Autodesk Inventor part; units mm, degrees
ref_plane "YZ Plane" through (0, 0, 0) normal (1, 0, 0) x (0, 1, 0)
ref_plane "XZ Plane" through (0, 0, 0) normal (0, 1, 0) x (-1, 0, 0)
ref_plane "XY Plane" through (0, 0, 0) normal (0, 0, 1) x (1, 0, 0)
sketch "Sketch3" plane through (0, 0, 0) normal (0, 0, 1) x (1, 0, 0)
  line L0 (735, 1100) -> (735, 35.3553)
  line L1 (735, 35.3553) -> (699.6447, 0)
  line L2 (699.6447, 0) -> (-699.6447, 0)
  line L3 (-699.6447, 0) -> (-735, 35.3553)
  line L4 (-735, 35.3553) -> (-735, 1100)
  line L5 (-735, 1100) -> (735, 1100)
  line L6 (0, 0) -> (0, 1100) construction
  line L7 (675, 1100) -> (584.0074, 850)
  line L8 (584.0074, 850) -> (159.0074, 850)
  line L9 (159.0074, 850) -> (68.0149, 1100)
  line L10 (-68.0149, 1100) -> (-159.0074, 850)
  line L11 (-159.0074, 850) -> (-584.0074, 850)
  line L12 (-584.0074, 850) -> (-675, 1100)
  line L13 (-735, 35.3553) -> (-735, 0)
  line L14 (-735, 0) -> (-699.6447, 0)
  line L15 (699.6447, 0) -> (735, 0)
  line L16 (735, 0) -> (735, 35.3553)
  dimension "d25" = 50
  dimension "d26" = 1100
  dimension "d27" = 1470
  dimension "d32" = 425
  dimension "d33" = 60
  dimension "d35" = 250
  dimension "d38" = 110
extrude "Plate3" add sketch "Sketch3" along normal blind 2 contours L0 L1 L2 L3 L4 L5 L12 L11 L10 L9 L8 L7 | L16 L15 L1 | L14 L13 L3
equation "\"d28\" = Thickness"
equation "\"BendRadius\" = Thickness"
equation "\"BendReliefWidth\" = Thickness"
equation "\"BendReliefDepth\" = 0.5 * Thickness"
equation "\"CornerReliefSize\" = 4 * Thickness"
equation "\"MinimumRemnant\" = 2 * Thickness"
equation "\"TransitionRadius\" = BendRadius"
equation "\"JacobiRadiusSize\" = BendRadius"
equation "\"GapSize\" = Thickness"
properties part number "GBK-RK-0015 partition 5"
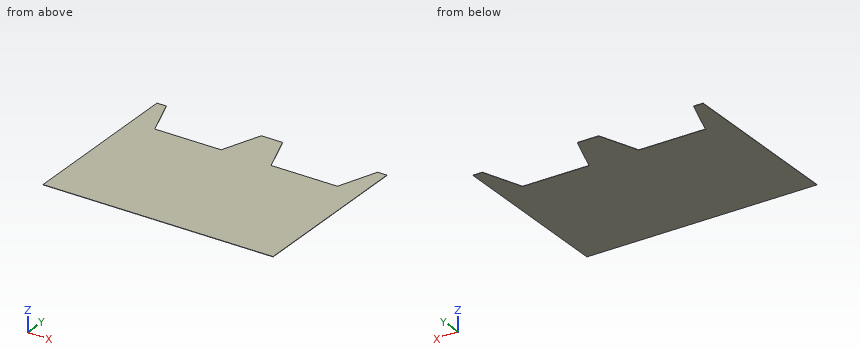
The listing builds one solid part. Answer for the finished solid, in the listing's coordinates (mm). Coordinates: 2 decimals unless noted, no trailing zeros. Write each loop counter-clockwise with the first axis right and the second up, starting at its lowest first coordinate (ties: lowest second). Pieces come first, ordered by that corner, then holes. Notation, with made-up numbers: (53.5, 18.25) - (107.5, 18.25) arc R17 cw to (107.5, 31.25) - close; hole circle Ø1 at (77.25, 60). An arc over 180 degrees is marked (long way). Return JSON: item names as keys, results as strings. Group by question number.
1. A cutting plane is placed at C-C, the plane x = 238. Determine the outline of the cut face in (y, z).
2. Given pin 1 (0.6 mm diameter, centred on x = 321.5, z = 0.5, fed in from +Y), flat-ended and moving along its own axis, determine where the tip first touches the part or whether it passes through.
3. Straight lines are drawn through the part: L1, parallel to X at y = 999, z = 1.4; L2, parallel to X at y = 902.5, z = 1.4; L3, parallel to Y at x = 339, z = 1.5. For each, find the intervals that lie inside material, in ascending order.
4. A cutting plane is placed at A-A, the plane z = 0.7. Determine the outline of the cut face in (x, y), plus the area to 3 significant figures.
5. A cutting plane is placed at B-B, the plane y = 872.5. Determine the outline of the cut face in (x, z).
Ans:
{
 "1": {"outline": "(0, 0) - (850, 0) - (850, 2) - (0, 2) - close"},
 "2": {"pin 1": "y = 850"},
 "3": {"L1": "-735 to -638.24, -104.78 to 104.78, 638.24 to 735", "L2": "-735 to -603.12, -139.9 to 139.9, 603.12 to 735", "L3": "0 to 850"},
 "4": {"outline": "(-735, 0) - (735, 0) - (735, 1100) - (675, 1100) - (584.01, 850) - (159.01, 850) - (68.01, 1100) - (-68.01, 1100) - (-159.01, 850) - (-584.01, 850) - (-675, 1100) - (-735, 1100) - close", "area": "1,360,000 mm²"},
 "5": {"outline": "(-735, 0) - (-592.2, 0) - (-592.2, 2) - (-735, 2) - close; (-150.82, 0) - (150.82, 0) - (150.82, 2) - (-150.82, 2) - close; (592.2, 0) - (735, 0) - (735, 2) - (592.2, 2) - close"}
}
